The model under review builds one solid part; all positions refer to its coordinate system, in mm. A direction names the side the tool comes from. Coordinates: 2 decimals unless noted, no trailing zeros. Loops run counter-clockwise (first coordinate to the right, second up) from the corner with the lowest first, then second, coordinate; pieces in that order, holes last. Notation, with made-up numbers: (54.25, 77) - (59.25, 77) arc R15 ccw to (59.25, 94) - close; hole circle Ø6 at (34.5, -6). An arc over 180 degrees is marked (long way). One line per item, written item: value. Start each with the question number.
1. We need section D-D, the plane x = -29. Give the boundary of the cut face in (y, z).
2. We need section A-A, the plane x = 12. Give the boundary of the cut face in (y, z), then the cut area to 3 significant figures.
3. For faces 1 (the face through (0, 75.07, -1.06)), 2 (the face through (30.07, 15, -1.06)), 3 (the face through (30.07, 75, -1.06)), 4 (the face through (37, 79.07, 5.58)), 5 (the face through (-0.07, 15, -1.06)), list the 3-axis set-ups (+Z, -Z, +X, -X, +Y, -Y) from which the entire face can be reached by the end or side of a thin tool; tool diameter is ignored.
4. Insertion check: P1, Ø2, axis at y = 79, z = 10.5, coming from the -X side; P2, Ø0.6, axis at y = 79, z = 10, coming from the +X side; P3, Ø1, axis at x = 17, z = -1, coming from the +Y side. Each pin has a flat end and moves straight along its axis. Give the tip position at first contact, or say it passes through.
5. To check wall thickness, follow line 1 (Z direction, x = -8, y = -15); line 2 (X direction, y = 14.5, z = -1); line 3 (Y direction, x = -0.5, z = -0.75). State the ranges of each line that lie inside material, in increasing order.
6. We need section B-B, the plane y = -37. Give the boundary of the cut face in (x, z), then the cut area to 3 significant figures.
7. We need section C-C, the plane x = 30. Give the boundary of the cut face in (y, z), then the cut area to 3 significant figures.
from build123d import *

# Parameters (mm, degrees)
SKETCH_1_W          = 77
SKETCH_1_H          = 161
EXTRUDE_1_DEPTH     = 11
SKETCH_2_W          = 33
SKETCH_2_H          = 63
EXTRUDE_2_DEPTH     = 2.1
FILLET_1_R          = 5
FILLET_2_R          = 5
SKETCH_3_W          = 32
SKETCH_3_H          = 2
CUT_EXTRUDE_1_DEPTH = 2
WRAP_1_OUTLINE_R    = 1
WRAP_1_DEPTH        = 0.01


# Read off the part's stored shape, not the designer's step: 包覆1
with BuildPart() as part:
    # 草图1 → 凸台-拉伸1 (new body)
    with BuildSketch(Plane.XY):
        Rectangle(SKETCH_1_W, SKETCH_1_H)
    extrude(amount=EXTRUDE_1_DEPTH)

    # 草图2 → 凸台-拉伸2 (add)
    with BuildSketch(Plane(origin=(0, 0, 0), x_dir=(-1, 0, 0), z_dir=(0, 0, -1))):
        with Locations((-15, 45)):
            Rectangle(SKETCH_2_W, SKETCH_2_H)
    extrude(amount=EXTRUDE_2_DEPTH)

    # 圆角1
    fillet_1_edges = [part.edges().sort_by_distance(p)[0] for p in [
        (31.5, 76.5, -1.05),
        (31.5, 13.5, -1.05),
        (-1.5, 13.5, -1.05),
        (-1.5, 76.5, -1.05),
    ]]
    fillet(fillet_1_edges, radius=FILLET_1_R)

    # 圆角2
    fillet_2_edges = [part.edges().sort_by_distance(p)[0] for p in [
        (38.5, -80.5, 5.5),
        (-38.5, -80.5, 5.5),
        (-38.5, 80.5, 5.5),
        (38.5, 80.5, 5.5),
    ]]
    fillet(fillet_2_edges, radius=FILLET_2_R)

    # 草图3 → 切除-拉伸1 (cut)
    with BuildSketch(Plane.XY.offset(11)):
        with Locations((0, 79)):
            Rectangle(SKETCH_3_W, SKETCH_3_H)
    extrude(amount=-CUT_EXTRUDE_1_DEPTH, mode=Mode.SUBTRACT)

    # 包覆1 outline → 包覆1 (add)
    with BuildSketch(Plane(origin=(0, 0, 0), x_dir=(-1, 0, 0), z_dir=(0, 0, -1))):
        Circle(WRAP_1_OUTLINE_R)
    extrude(amount=WRAP_1_DEPTH)


solid = part.part
Findings below:
1. outline: (-80.5, 0) - (80.5, 0) - (80.5, 11) - (-80.5, 11) - close
2. outline: (-80.5, 0) - (13.5, 0) - (13.5, -2.1) - (76.5, -2.1) - (76.5, 0) - (80.5, 0) - (80.5, 11) - (80, 11) - (80, 9) - (78, 9) - (78, 11) - (-80.5, 11) - close
2. area: 1,900 mm2
3. face 1: -Z, -X, +Y
3. face 2: -Z, +X, -Y
3. face 3: -Z, +X, +Y
3. face 4: +Z, -Z, +X, +Y
3. face 5: -Z, -X, -Y
4. P1: x = -37.83
4. P2: x = 37.34
4. P3: y = 76.5
5. line 1: 0 to 11
5. line 2: 0.5 to 29.5
5. line 3: 15.5 to 74.5
6. outline: (-38.5, 0) - (38.5, 0) - (38.5, 11) - (-38.5, 11) - close
6. area: 847 mm2
7. outline: (-80.5, 0) - (14.93, 0) - (14.93, -2.1) - (75.07, -2.1) - (75.07, 0) - (80.5, 0) - (80.5, 11) - (-80.5, 11) - close
7. area: 1,900 mm2
